Work out the finished part from the listing and answer in its coordinate system (mm). Face numbers are marked on the shaded views. A direction names the side the tool comes from. Coordinates: 2 decimals unless noted, no trailing zeros. Order: outer loops, then holes, each group sorted by start corner. A loop starts at its lowest first (then second) coordinate and runs counter-clockwise, first axis right, second up. Notation, with made-up numbers: M -19,0 L 27,0 A22 cw 27,15 Z; hole C 50.5,41 d6. An arc over 180 degrees is marked long. Answer in a Markdown table with one row per item. Add a question column.
Item 1: Consider line 1 (Z direction, x = -55, y = 62); line 2 (Y direction, x = 25, z = -27); line 3 (Y direction, x = 47.5, z = -18.5). Determine where each line is inside the solid, lowest interval first. Write a range as from..to.
Item 2: Which of the six approach directions +Z, -Z, +X, -X, +Y, -Y give full straight-line access (tool end or side, diameter ignored) to the marked faces 1, 2 and 3?
Item 3: The part is cut by section A-A (x = 55). Write down the section's boundary in (y, z), then the cut area to 3 significant figures.
Item 4: The part is cut by section B-B (z = -15). Write down the section's boundary in (x, y), then the cut area to 3 significant figures.
Item 5: The part is cut by section D-D (z = -63). Write down the section's boundary in (x, y) (3 decimals), then the cut area to 3 significant figures.
Item 6: Flat-ended cylindrical pins translate along their axes: pin 1 Ø15 at (x, y) = (-58.5, 38) entering from +Z; pin 2 Ø6 at (x, y) = (-3.5, 26) entering from -Z; pin 3 Ø9 at (x, z) = (-61.5, -20) entering from -Y. Find the tip coordinate at first contact, or state that the pin passes through.
Item 7: The part is cut by section C-C (y = 35). Write down the section's boundary in (x, z).
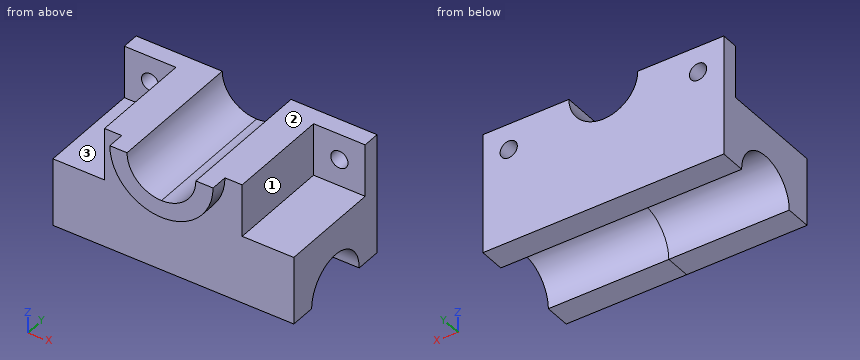
from build123d import *
from build123d import SkipClean  # not in build123d's __all__

# Parameters (mm, degrees)
F1_DEPTH = 70
F2_W     = 30
F2_H     = 30.5260747812
F3_DEPTH = 60
F4_R     = 5
F5_DEPTH = 10.001
F6_R     = 20
F7_DEPTH = 70.001
F9_DEPTH = 10


with BuildPart() as f1:
    # F0 (on Front) → F1 (new body)
    with BuildSketch(Plane.XZ):
        with BuildLine():
            Line((0, -20), (0, -70))
            Line((0, -70), (70, -70))
            Line((70, -70), (70, 0))
            Line((70, 0), (20, 0))
            ThreePointArc((20, 0), (14.1421356237, -14.1421356237), (0, -20))
        make_face()
    extrude(amount=-F1_DEPTH)

    # F2 (on face) → F3 (cut)
    with BuildSketch(Plane.XZ):
        with Locations((55, -15.2630373906)):
            Rectangle(F2_W, F2_H)
    extrude(amount=-F3_DEPTH, mode=Mode.SUBTRACT)

    # F4 (on face) → F5 (cut, through all)
    with BuildSketch(Plane.XZ.offset(-60)):
        with Locations((55, -15)):
            Circle(F4_R)
    extrude(amount=-F5_DEPTH, mode=Mode.SUBTRACT)

    # F6 (on face) → F7 (cut, through all)
    with BuildSketch(Plane.YZ.offset(70)):
        with Locations((35, -70)):
            Circle(F6_R)
    extrude(amount=-F7_DEPTH, mode=Mode.SUBTRACT)

    # F8 (on face) → F9 (join)
    with BuildSketch(Plane.XZ):
        with BuildLine():
            ThreePointArc((20, 0), (14.1421356237, -14.1421356237), (0, -20))
            Line((0, -20), (0, -30))
            ThreePointArc((0, -30), (21.2132034356, -21.2132034356), (30, 0))
            Line((30, 0), (20, 0))
        make_face()
    extrude(amount=F9_DEPTH)

    # F10: F1 across plane


with BuildPart() as f1_1:
    add(f1.part, clean=False)
    with SkipClean():  # cleaning this boolean's faces spoils the solid; the shape is the same uncleaned
        add(f1.part.mirror(Plane.YZ), clean=False)


solid = f1_1.part
Reply:
| question | item | result |
|---|---|---|
| 1 | line 1 | z = -70..-20, -10..0 |
| 1 | line 2 | y = 0..70 |
| 1 | line 3 | y = 60..70 |
| 2 | face 1 | +Z, +X, -Y |
| 2 | face 2 | +Z, +X, -X, +Y, -Y |
| 2 | face 3 | +Z, -X, -Y |
| 3 | outline | M 0,-70 L 15,-70 A20 cw 55,-70 L 70,-70 L 70,-20 L 60,-20 L 60,-30.53 L 0,-30.53 Z; M 60,-10 L 70,-10 L 70,0 L 60,0 Z |
| 3 | area | 2,340 mm2 |
| 4 | outline | M -70,60 L -60,60 L -60,70 L -70,70 Z; M -50,60 L -40,60 L -40,0 L -25.98,0 L -25.98,-10 L -13.23,-10 L -13.23,70 L -50,70 Z; M 13.23,-10 L 25.98,-10 L 25.98,0 L 40,0 L 40,60 L 50,60 L 50,70 L 13.23,70 Z; M 60,60 L 70,60 L 70,70 L 60,70 Z |
| 4 | area | 4,400 mm2 |
| 5 | outline | M -70,0 L 70,0 L 70,16.265 L -70,16.265 Z; M -70,53.735 L 70,53.735 L 70,70 L -70,70 Z |
| 5 | area | 4,550 mm2 |
| 6 | pin 1 | stops at z = -30.53 |
| 6 | pin 2 | stops at z = -54 |
| 6 | pin 3 | stops at y = 60 |
| 7 | outline | M -70,-50 L 70,-50 L 70,-30.53 L 40,-30.53 L 40,0 L 20,0 A20 cw -20,0 L -40,0 L -40,-30.53 L -70,-30.53 Z |
